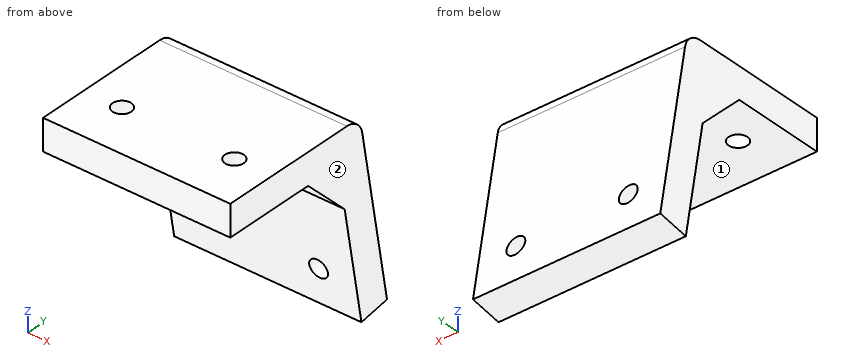
```python
from build123d import *

# Parameters (mm, degrees)
EXTRUDE_1_DEPTH     = 30
FILLET_1_R          = 3
SKETCH_2_R          = 1.5
CUT_EXTRUDE_1_DEPTH = 53.32140222
SKETCH_3_R          = 1.5
CUT_EXTRUDE_2_DEPTH = 52.875952527
EXTRUDE_2_DEPTH     = 30


with BuildPart() as part:
    # 草图1 → 凸台-拉伸1 (new body)
    with BuildSketch(Plane(origin=(0, 0, 0), x_dir=(0, 0, -1), z_dir=(1, 0, 0))):
        Polygon((0, 0), (5, 0), (5, 20.804501844), (30.412473479, 25.285406565), (29.54423259, 30.20944533), (0, 25), align=None)
    extrude(amount=EXTRUDE_1_DEPTH)

    # 圆角1
    fillet_1_edges = [part.edges().sort_by_distance(p)[0] for p in [
        (15, 25, 0),
        (15, 20.804501844, -5),
    ]]
    fillet(fillet_1_edges, radius=FILLET_1_R)

    # 草图2 → 切除-拉伸1 (cut, through all)
    with BuildSketch(Plane.XY):
        with Locations((6, 8)):
            Circle(SKETCH_2_R)
        with Locations((24, 8)):
            Circle(SKETCH_2_R)
    extrude(amount=-CUT_EXTRUDE_1_DEPTH, mode=Mode.SUBTRACT)

    # 草图3 → 切除-拉伸2 (cut, through all)
    with BuildSketch(Plane(origin=(0, 24.24615776, 4.275251792), x_dir=(1, 0, 0), z_dir=(0, 0.9848077530122086, 0.1736481776669273))):
        with Locations(Location((6, 28.341204442, 0), (0, 0, 270))):
            Circle(SKETCH_3_R)
        with Locations(Location((24, 28.341204442, 0), (0, 0, 270))):
            Circle(SKETCH_3_R)
    extrude(amount=-CUT_EXTRUDE_2_DEPTH, mode=Mode.SUBTRACT)

    # 草图4 → 凸台-拉伸2 (add)
    with BuildSketch(Plane(origin=(30, 0, 0), x_dir=(0, 0, -1), z_dir=(1, 0, 0))):
        with BuildLine():
            Line((5, 15), (5, 18.287202951))
            ThreePointArc((5, 18.287202951), (5.701866671, 20.21556578), (7.479055467, 21.24162621))
            Line((7.479055467, 21.24162621), (12.047094791, 22.047094791))
            Line((12.047094791, 22.047094791), (5, 15))
        make_face()
    extrude(amount=-EXTRUDE_2_DEPTH)


solid = part.part
```
Design review of the part built by this model. Coordinates are the model's own, in mm. Face numbers are marked on the shaded views. A direction names the side the tool comes from. Give positions to 0.01 mm unless a question says otherwise; leave off trailing zeros. Write each loop counter-clockwise with the first axis right and the second up, starting at its lowest first coordinate (ties: lowest second). Pieces come first, ordered by that corner, then holes. Notation, with made-up numbers: (30.25, -15) -> (60.25, -15) arc R34 cw to (60.25, 19) -> close; hole circle Ø3 at (25.25, -34). An arc over 180 degrees is marked (long way). Answer in a Markdown table with one row per item.
(1) For the marked faces 1 and 2, list the 3-axis set-ups (+Z, -Z, +X, -X, +Y, -Y) from which the entire face can be reached by the end or side of a thin tool; tool diameter is ignored.
Results:
| item | result |
|---|---|
| face 1 | -Z, +X, -X, -Y |
| face 2 | +Z, -Z, +X, +Y, -Y |
(2) To check wall thickness, follow probe 1 along Y at (x, z) = (24, -2.8); probe 2 along Z at (x, y) = (18.5, 4.5); probe 3 along Y at (x, z) = (24, -1.15). State the ranges of each line that lie inside material, in increasing order.
Results:
| item | result |
|---|---|
| probe 1 | 0 to 6.5, 9.5 to 25.49 |
| probe 2 | -5 to 0 |
| probe 3 | 0 to 6.5, 9.5 to 24.84 |
(3) Consider section D-D (y = 27). Count the separate pieces of the cut face and the enclosed holes in it, then the cut area to 3 significant figures.
Results:
| item | result |
|---|---|
| separate pieces | 1 |
| enclosed holes | 2 |
| area | 549 mm2 |
(4) Consider section C-C (z = -4). State the section outline as (x, y) points.
Results:
| item | result |
|---|---|
| outline | (0, 0) -> (30, 0) -> (30, 25.71) -> (0, 25.71) -> close; hole circle Ø3 at (6, 8); hole circle Ø3 at (24, 8) |
(5) Consider section A-A (y = 8). State the section outline as (x, z) points, then the cut area to 3 significant figures.
Results:
| item | result |
|---|---|
| outline | (0, -5) -> (4.5, -5) -> (4.5, 0) -> (0, 0) -> close; (7.5, -5) -> (22.5, -5) -> (22.5, 0) -> (7.5, 0) -> close; (25.5, -5) -> (30, -5) -> (30, 0) -> (25.5, 0) -> close |
| area | 120 mm2 |
(6) Clearance check with flat-ended pins moving along their axes: pin 1 (7.5 mm diameter, centred on x = 13, y = 11, fed in from -Z); pin 2 (1.5 mm diameter, centred on x = 26, z = -5.5, fed in from +Y); pin 3 (5 mm diameter, centred on x = 16, z = -6, fed in from -Y); pin 4 (4 mm diameter, centred on x = 25.5, z = -9, fed in from -Y). State where each tip first meets the part, or that it passes through.
Results:
| item | result |
|---|---|
| pin 1 | z = -5 |
| pin 2 | y = 26.1 |
| pin 3 | y = 0 |
| pin 4 | y = 17 |
(7) Consider section B-B (x = 21.5). State the section outline as (y, z) points, then the cut area to 3 significant figures.
Results:
| item | result |
|---|---|
| outline | (0, -5) -> (15, -5) -> (22.05, -12.05) -> (25.29, -30.41) -> (30.21, -29.54) -> (25.44, -2.48) arc R3 ccw to (22.48, 0) -> (0, 0) -> close |
| area | 273 mm2 |
